```python
from build123d import *

# Parameters (mm, degrees)
F1_DEPTH = 100
F2_W     = 38.2318552583
F2_H     = 21.9314545393
F3_DEPTH = 37.5
F4_W     = 31.1708524823
F4_H     = 11.4039704204
F5_DEPTH = 100
F6_R     = 7.2110189045
F6_R_2   = 9.4884997303
F6_R_3   = 8.9600155303
F6_R_4   = 7.162126067
F7_DEPTH = 2500


with BuildPart() as f1:
    # F0 (on Front) → F1 (new body)
    with BuildSketch(Plane.XZ):
        Polygon((-49.1552427411, 37.2157283127), (-49.1552427411, 0), (0, 0), (0, -12.0665328577), (52.7116954327, -12.0665328577), (0, 37.2157283127), align=None)
    extrude(amount=F1_DEPTH)

    # F2 (on Top) → F3 (cut, symmetric)
    with BuildSketch(Plane.XY):
        with Locations((36.1572587863, -89.4082635641)):
            Rectangle(F2_W, F2_H)
    extrude(amount=F3_DEPTH, both=True, mode=Mode.SUBTRACT)

    # F4 (on Right) → F5 (cut, symmetric)
    with BuildSketch(Plane.YZ):
        with Locations((-50.8213154972, 34.0540632606)):
            Rectangle(F4_W, F4_H)
    extrude(amount=F5_DEPTH, both=True, mode=Mode.SUBTRACT)

    # F6 (on Top) → F7 (cut, symmetric)
    with BuildSketch(Plane.XY):
        with Locations((13.7812495232, -60.6602802873)):
            Circle(F6_R)
        with Locations((36.6018153727, -59.4747960567)):
            Circle(F6_R_2)
        with Locations((33.9344777167, -21.5393137187)):
            Circle(F6_R_3)
        with Locations((12.595766224, -26.5776216984)):
            Circle(F6_R_4)
    extrude(amount=F7_DEPTH, both=True, mode=Mode.SUBTRACT)


solid = f1.part
```
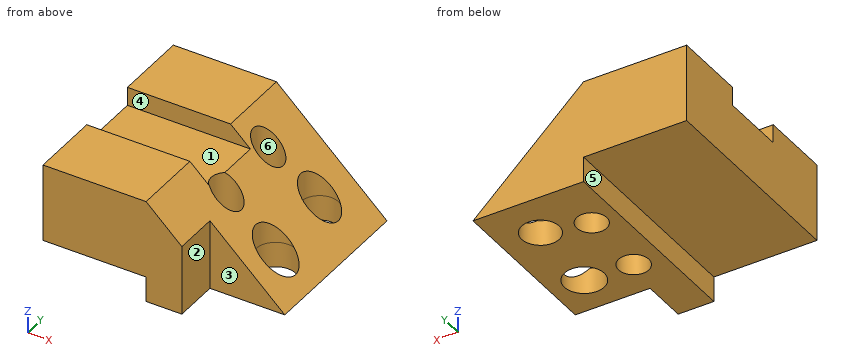
CAD build for the part. Positions are in the model's coordinates, mm. Face numbers are marked on the shaded views. A direction names the side the tool comes from. Give positions to 0.01 mm unless a question says otherwise; leave off trailing zeros. Order: outer loops, then holes, each group sorted by start corner. A loop starts at its lowest first (then second) coordinate and runs counter-clockwise, first axis right, second up. Notation, with made-up numbers: M 71.25,57.25 L 129.25,57.25 A19 cw 129.25,81.25 Z; hole C 13.5,-30 d1. An arc over 180 degrees is marked long. Put each result on its own line as item: value. Start each with the question number.
(1) Saw through at B-B, the plane z = 8. Write the cut outline in (x, y).
(2) Mould opens along Y. For the marked faces 1, 2 and 3 say: +Y half, -Y half, draft (parallel to the pull), parting line (faces both ways), or undercut.
(3) Flat gauge pins, fed straight in: pin 1 Ø10 at (x, y) = (-32.5, -45.5) entering from -Z; pin 2 Ø3.5 at (y, z) = (-33, -3.5) entering from -X; pin 3 Ø23.5 at (y, z) = (-93.5, 9) entering from +X; pin 4 Ø18.5 at (x, y) = (13.78, -60.66) entering from -Z. Where does each tip first touch, or does it go through?
(4) Which spindle directions (+Z, -Z, +X, -X, +Y, -Y) get a long thin tool onto all of the face, cutting with end or side? Do the marked faces 4, 5 and 6. Say none if no direction does.
(5) Saw through at C-C, the plane y = -16. Write the cut outline in (x, z), then the cut area to 3 significant figures.
(6) Saw through at A-A, the plane y = -92. Write the cut outline in (x, z).
(7) Saw through at D-D, the plane x = -16. Write the cut outline in (y, z).
(8) Drill centre lines: line 1 along Y through (x, z) = (17.5, 15.5); line 2 along Y through (x, z) = (38, -2.5); line 3 along Y through (x, z) = (-18.5, 32). Where is each one in solid material? Low to high.
Check result:
1. outline: M -49.16,-100 L 17.04,-100 L 17.04,-78.44 L 31.25,-78.44 L 31.25,-67.31 A9.49 cw 31.25,-51.64 L 31.25,-30.09 A8.96 cw 31.25,-12.99 L 31.25,0 L -49.16,0 Z; hole C 12.6,-26.58 d14.32; hole C 13.78,-60.66 d14.42
2. face 1: undercut
2. face 2: draft
2. face 3: -Y half
3. pin 1: stops at z = 0
3. pin 2: stops at x = 0
3. pin 3: stops at x = 17.04
3. pin 4: stops at z = -12.07
4. face 4: +Z, +X, -X
4. face 5: -Z, -X, +Y, -Y
4. face 6: +Z, -Z
5. outline: M -49.16,0 L 0,0 L 0,-12.07 L 26.89,-12.07 L 26.89,12.07 L 0,37.22 L -49.16,37.22 Z; M 40.98,-12.07 L 52.71,-12.07 L 40.98,-1.1 Z
5. area: 2,880 mm2
6. outline: M -49.16,0 L 0,0 L 0,-12.07 L 17.04,-12.07 L 17.04,21.28 L 0,37.22 L -49.16,37.22 Z
7. outline: M -100,0 L 0,0 L 0,37.22 L -35.24,37.22 L -35.24,28.35 L -66.41,28.35 L -66.41,37.22 L -100,37.22 Z
8. line 1: y = -78.44 to -66.84, -54.48 to -31.8, -21.36 to 0
8. line 2: y = -78.44 to -68.86, -50.09 to -29.52, -13.55 to 0
8. line 3: y = -100 to -66.41, -35.24 to 0
